Autodesk Inventor part; units mm, degrees
ref_plane "YZ Plane" through (0, 0, 0) normal (1, 0, 0) x (0, 1, 0)
ref_plane "XZ Plane" through (0, 0, 0) normal (0, 1, 0) x (-1, 0, 0)
ref_plane "XY Plane" through (0, 0, 0) normal (0, 0, 1) x (1, 0, 0)
sketch "Sketch1" plane through (0, 0, 0) normal (0, 1, 0) x (-1, 0, 0)
  line L0 (7.3612, -4.25) -> (0, -8.5)
  line L1 (0, -8.5) -> (-7.3612, -4.25)
  line L2 (-7.3612, -4.25) -> (-7.3612, 4.25)
  line L3 (-7.3612, 4.25) -> (0, 8.5)
  line L4 (0, 8.5) -> (7.3612, 4.25)
  line L5 (7.3612, 4.25) -> (7.3612, -4.25)
  line L6 (15.3979, -8.89) -> (0, -17.78)
  line L7 (0, -17.78) -> (-15.3979, -8.89)
  line L8 (-15.3979, -8.89) -> (-15.3979, 8.89)
  line L9 (-15.3979, 8.89) -> (0, 17.78)
  line L10 (0, 17.78) -> (15.3979, 8.89)
  line L11 (15.3979, 8.89) -> (15.3979, -8.89)
  point P0 (0, 0)
  point P1 (0, 0)
  point P2 (0, 0)
  dimension "d0" = 8.5
  dimension "d1" = 17.78
extrude "Extrusion1" add sketch "Sketch1" along normal blind 6.35
fillet "Fillet1" radius 3.175 6 edges at (-15.3979, 3.175, 8.89) (0, 3.175, 17.78) (15.3979, 3.175, 8.89) (15.3979, 3.175, -8.89) (0, 3.175, -17.78) (-15.3979, 3.175, -8.89)
properties part number "Bolt Head_3DPrint"
Design review of the part built by this model. Coordinates are the model's own, in mm. A direction names the side the tool comes from. Coordinates: 2 decimals unless noted, no trailing zeros. Order: outer loops, then holes, each group sorted by start corner. A loop starts at its lowest first (then second) coordinate and runs counter-clockwise, first axis right, second up. Notation, with made-up numbers: M 79,89.25 L 86,89.25 A20 ccw 86,117.25 Z; hole C -18.5,5 d7. An arc over 180 degrees is marked long. Answer as a JSON object with one key per item and string values. Group by question number.
1) Add section C-C, the plane x = -2. Write out the cut boundary in (y, z).
2) Add section D-D, the plane z = -13.5. Write out the cut boundary in (x, y), then the cut area to 3 significant figures.
3) Wall thickness on L1, parallel to X at y = 1, z = -1; L2, parallel to Z at x = -3.5, y = 2.75; L3, parallel to Z at x = 5, y = 5.75: over which ranges is each line inside the solid? List them lowest first.
4) Mouldability with a two-part tool opening along X and no side actions: class faces 3 (the flat face through (3.629, 3.131, -6.405)), 4 (the flat face through (7.613, 3.131, -13.384)), 5 (the flat face through (-7.613, 3.131, 13.384)) as pulls with the +X half, pulls with the -X half, needs draft (parallel to the pull), parting line crosses it, or undercut.
5) For pin 1 (1.5 mm diameter, centred on y = 2, z = -12.5, fed in from -X), flat-tipped, find the tip position at first contact; note if it passes through.
6) Add section A-A, the plane z = -3.5. Write out the cut boundary in (x, y).
7) Tool access review of faces 1 (the cylindrical face through (0.02, 3.22, -17.29)), 2 (the flat face through (7.361, 3, 0)): name each direction out of +Z, -Z, +X, -X, +Y, -Y from which nothing blocks a thin tool from reaching the whole face with its end or side.
Computed values:
{
 "1": {"outline": "M 0,-16.63 L 6.35,-16.63 L 6.35,-7.35 L 0,-7.35 Z; M 0,7.35 L 6.35,7.35 L 6.35,16.63 L 0,16.63 Z"},
 "2": {"outline": "M -7.41,0 L 7.41,0 L 7.41,6.35 L -7.41,6.35 Z", "area": "94.1 mm^2"},
 "3": {"L1": "x = -15.4 to -7.36, 7.36 to 15.4", "L2": "z = -15.76 to -6.48, 6.48 to 15.76", "L3": "z = -14.89 to -5.61, 5.61 to 14.89"},
 "4": {"face 3": "undercut", "face 4": "pulls with the +X half", "face 5": "pulls with the -X half"},
 "5": {"pin 1": "stops at x = -10.44"},
 "6": {"outline": "M -15.4,0 L -7.36,0 L -7.36,6.35 L -15.4,6.35 Z; M 7.36,0 L 15.4,0 L 15.4,6.35 L 7.36,6.35 Z"},
 "7": {"face 1": "-Z, +Y, -Y", "face 2": "+Y, -Y"}
}
